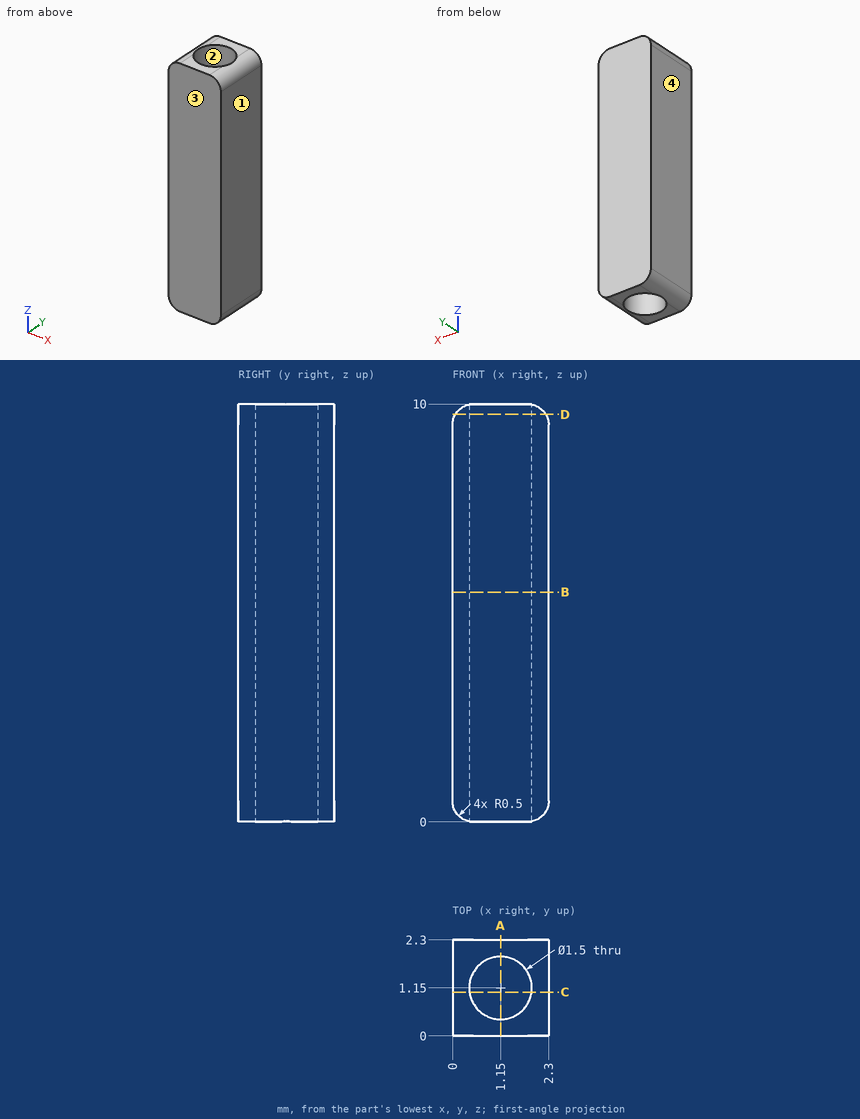
Here's the drawing with two shaded views (mm, measured from the low corner). I have some questions. Round coordinates to 2 decimals unless told otherwise and drop trailing zeros. Order: outer loops, then holes, each group sorted by start corner. A loop starts at its lowest first (then second) coordinate and runs counter-clockwise, first axis right, second up. Notation, with made-up numbers: (33.5, 62.25) -> (46.5, 62.25) arc R20 cw to (46.5, 97.25) -> close; hole circle Ø6 at (85.25, 78.25). An arc over 180 degrees is marked (long way). Use a Markdown table: item, result. Add a question column.
(1) Suppose I cut it at D-D, the plane z = 9.75. Please give me the cut outline in (x, y), and give its area (3 significant figures).
(2) If we mould it in two halves opening along X, with no side actions, what happens to the marked faces 1, 2, 3 and 4? For each: released by +X, released by -X, zero draft, split by the parting line, or undercut.
(3) Suppose I cut it at A-A, the plane x = 1.15. Please give me the cut outline in (y, z).
(4) Suppose I cut it at B-B, the plane z = 5.5. Please give me the cut outline in (x, y), and give its area (3 significant figures).
(5) Suppose I cut it at C-C, the plane y = 1.05. Please give me the cut outline in (x, z).
(6) I need wall thicknesses on line 1 along Y through (x, z) = (1.5, 4.75); line 2 along X through (y, z) = (1.65, 5); line 3 along X through (y, z) = (1.75, 3.5). Which ranges of each line are inside material? Lowest first, please.
Verdict:
| question | item | result |
|---|---|---|
| 1 | outline | (0.07, 0) -> (2.23, 0) -> (2.23, 2.3) -> (0.07, 2.3) -> close; hole circle Ø1.5 at (1.15, 1.15) |
| 1 | area | 3.21 mm2 |
| 2 | face 1 | released by +X |
| 2 | face 2 | undercut |
| 2 | face 3 | zero draft |
| 2 | face 4 | released by -X |
| 3 | outline | (0, 0) -> (0.4, 0) -> (0.4, 10) -> (0, 10) -> close; (1.9, 0) -> (2.3, 0) -> (2.3, 10) -> (1.9, 10) -> close |
| 4 | outline | (0, 0) -> (2.3, 0) -> (2.3, 2.3) -> (0, 2.3) -> close; hole circle Ø1.5 at (1.15, 1.15) |
| 4 | area | 3.52 mm2 |
| 5 | outline | (0, 0.5) arc R0.5 ccw to (0.41, 0.01) -> (0.41, 9.99) arc R0.5 ccw to (0, 9.5) -> close; (1.89, 0.01) arc R0.5 ccw to (2.3, 0.5) -> (2.3, 9.5) arc R0.5 ccw to (1.89, 9.99) -> close |
| 6 | line 1 | 0 to 0.49, 1.81 to 2.3 |
| 6 | line 2 | 0 to 0.59, 1.71 to 2.3 |
| 6 | line 3 | 0 to 0.7, 1.6 to 2.3 |
